Source: CAD feature listing. Evaluate the final solid. Frame: model axes, mm. Give positions to 0.01 mm unless a question says otherwise; leave off trailing zeros. Order: outer loops, then holes, each group sorted by start corner. A loop starts at its lowest first (then second) coordinate and runs counter-clockwise, first axis right, second up. Notation, with made-up numbers: M -10,42.5 L 24,42.5 A21 ccw 24,81.5 Z; hole C 43,76 d3. An arc over 180 degrees is marked long. Use CSV: the item, a comma, the result in double quotes. Start each with the question number.
1. Section query A-A, the plane z = -245. Return the cut outline in (x, y), plus the area to 3 significant figures.
2. Line query: line 1 along Z through (x, y) = (0, -3.5); line 2 along Z through (x, y) = (6, 2.5); line 3 along Y through (x, z) = (-5, 245). Output: solid intervals per line, ascending. Write a range as [from, to].
3. Pin query (flat end, axial travel): P1, Ø4, axis at y = -2.5, z = -245.5, coming from the +X side; P2, Ø4, axis at x = 1, z = -210, coming from the +Y side; P3, Ø5, axis at y = 0, z = -245, coming from the -X side. Return the tip coordinate at first contact, or that it passes through.
4. Section query B-B, the plane x = 1.75. State how many separate pieces and enclosed holes the cut face has, plus the area to 3 significant figures.
from build123d import *

# Parameters (mm, degrees)
IZIM1_W                     = 15
IZIM1_H                     = 15
Y_KSEKLIK_EKSTR_ZYON1_DEPTH = 252.5
DELIK2_D                    = 8.5
DELIK2_DEPTH                = 15
DELIK2_CBORE_D              = 14
DELIK2_CBORE_DEPTH          = 8
DELIK3_D                    = 8.5
DELIK3_DEPTH                = 15
DELIK3_CBORE_D              = 14
DELIK3_CBORE_DEPTH          = 8
L_O_ALTMA1_COUNT            = 3
L_O_ALTMA1_PITCH            = 212.5


with BuildPart() as part:
    # Çizim1 → Yükseklik-Ekstrüzyon1 (new body, symmetric)
    with BuildSketch(Plane.XY):
        Rectangle(IZIM1_W, IZIM1_H)
    extrude(amount=Y_KSEKLIK_EKSTR_ZYON1_DEPTH, both=True)

    # Delik2
    with Locations(Plane(origin=(7.5, 0, 0), x_dir=(0, 0, -1), z_dir=(1, 0, 0))):
        with Locations((245, 0)):
            delik2 = CounterBoreHole(DELIK2_D / 2, DELIK2_CBORE_D / 2, DELIK2_CBORE_DEPTH, depth=DELIK2_DEPTH)

    # Aynalama1: Delik2 across plane
    add(delik2.mirror(Plane.XY), mode=Mode.SUBTRACT)

    # Delik3
    with Locations(Plane(origin=(0, 7.5, 0), x_dir=(1, 0, 0), z_dir=(0, 1, 0))):
        with Locations((0, -212.5)):
            delik3 = CounterBoreHole(DELIK3_D / 2, DELIK3_CBORE_D / 2, DELIK3_CBORE_DEPTH, depth=DELIK3_DEPTH)

    # LÇoğaltma1: Delik3 ×3
    with Locations(*[(0, 0, -i * L_O_ALTMA1_PITCH) for i in range(1, L_O_ALTMA1_COUNT)]):
        add(delik3, mode=Mode.SUBTRACT)


solid = part.part
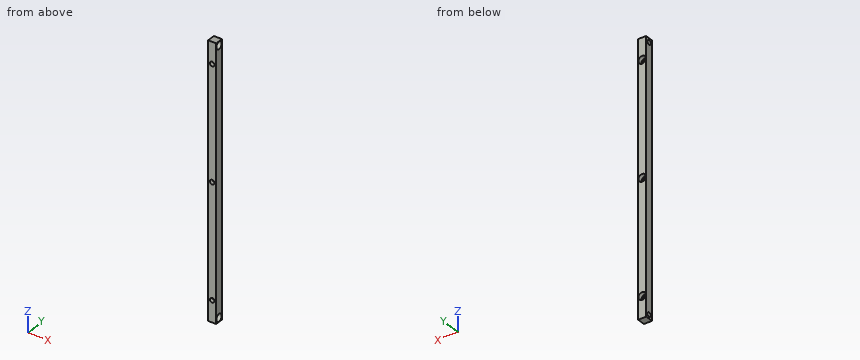
Result set:
1,outline,"M -7.5,-7.5 L 7.5,-7.5 L 7.5,-7 L -0.5,-7 L -0.5,-4.25 L -7.5,-4.25 Z; M -7.5,4.25 L -0.5,4.25 L -0.5,7 L 7.5,7 L 7.5,7.5 L -7.5,7.5 Z"
1,area,"53.5 mm2"
2,line 1,"[-252.5, -251.06], [-238.94, -216.75], [-208.25, -4.25], [4.25, 208.25], [216.75, 238.94], [251.06, 252.5]"
2,line 2,"[-252.5, -251.54], [-238.46, -216.11], [-208.89, -3.61], [3.61, 208.89], [216.11, 238.46], [251.54, 252.5]"
2,line 3,"[-7.5, -4.25], [4.25, 7.5]"
3,P1,"x = -0.5"
3,P2,"y = -0.5"
3,P3,"through"
4,separate pieces,"4"
4,enclosed holes,"2"
4,area,"6,780 mm2"
